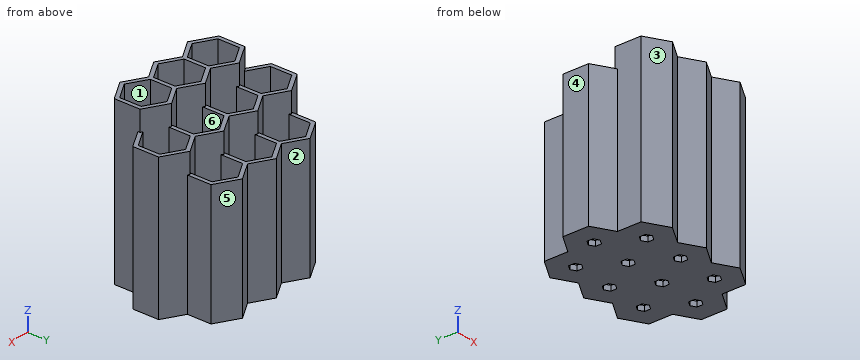
from build123d import *

# Parameters (mm, degrees)
F3_DEPTH = 101.6
F4_DEPTH = 88.9
F5_DEPTH = 76.2
F7_DEPTH = 3.175


with BuildPart() as f3:
    # F1 (on Top) → F3 (new body)
    with BuildSketch(Plane.XY):
        Polygon((0, -5.911706), (-12.620625, -13.198227), (-25.24125, -5.911706), (-39.0525, -13.885635), (-39.0525, -29.833493), (-25.24125, -37.807422), (-12.620625, -30.5209), (0, -37.807422), (12.620625, -30.5209), (25.24125, -37.807422), (39.0525, -29.833493), (39.0525, -13.885635), (25.24125, -5.911706), (12.620625, -13.198227), align=None)
        Polygon((0, -35.057791), (-11.43, -28.458677), (-11.43, -15.26045), (0, -8.661337), (11.43, -15.26045), (11.43, -28.458677), align=None, mode=Mode.SUBTRACT)
        Polygon((-25.24125, -35.057791), (-36.67125, -28.458677), (-36.67125, -15.26045), (-25.24125, -8.661337), (-13.81125, -15.26045), (-13.81125, -28.458677), align=None, mode=Mode.SUBTRACT)
        Polygon((13.81125, -28.458677), (13.81125, -15.26045), (25.24125, -8.661337), (36.67125, -15.26045), (36.67125, -28.458677), (25.24125, -35.057791), align=None, mode=Mode.SUBTRACT)
    extrude(amount=F3_DEPTH)

    # F0 (on Top) → F4 (join)
    with BuildSketch(Plane.XY):
        Polygon((-26.431875, -6.599114), (-24.050625, -6.599114), (-24.050625, 6.599114), (-12.620625, 13.198227), (-1.190625, 6.599114), (-1.190625, -6.599114), (1.190625, -6.599114), (1.190625, 6.599114), (12.620625, 13.198227), (24.050625, 6.599114), (24.050625, -6.599114), (26.431875, -6.599114), (26.431875, 6.599114), (37.861875, 13.198227), (49.291875, 6.599114), (49.291875, -6.599114), (37.861875, -13.198227), (39.0525, -15.26045), (51.673125, -7.973929), (51.673125, 7.973929), (37.861875, 15.947858), (25.24125, 8.661337), (12.620625, 15.947858), (0, 8.661337), (-12.620625, 15.947858), (-25.24125, 8.661337), (-37.861875, 15.947858), (-51.673125, 7.973929), (-51.673125, -7.973929), (-39.0525, -15.26045), (-37.861875, -13.198227), (-49.291875, -6.599114), (-49.291875, 6.599114), (-37.861875, 13.198227), (-26.431875, 6.599114), align=None)
    extrude(amount=F4_DEPTH)

    # F2 (on Top) → F5 (join)
    with BuildSketch(Plane.XY):
        Polygon((-13.81125, 15.26045), (-11.43, 15.26045), (-11.43, 28.458677), (0, 35.057791), (11.43, 28.458677), (11.43, 15.26045), (13.81125, 15.26045), (13.81125, 28.458677), (25.24125, 35.057791), (36.67125, 28.458677), (36.67125, 15.26045), (39.0525, 15.26045), (39.0525, 29.833493), (25.24125, 37.807422), (12.620625, 30.5209), (0, 37.807422), (-12.620625, 30.5209), (-25.24125, 37.807422), (-39.0525, 29.833493), (-39.0525, 15.26045), (-36.67125, 15.26045), (-36.67125, 28.458677), (-25.24125, 35.057791), (-13.81125, 28.458677), align=None)
    extrude(amount=F5_DEPTH)

    # F6 (on Top) → F7 (join)
    with BuildSketch(Plane.XY):
        Polygon((-49.291875, 6.599114), (-49.291875, -6.599114), (-37.861875, -13.198227), (-26.431875, -6.599114), (-26.431875, 6.599114), (-37.861875, 13.198227), align=None)
        Polygon((-37.861875, -3.666174), (-41.036875, -1.833087), (-41.036875, 1.833087), (-37.861875, 3.666174), (-34.686875, 1.833087), (-34.686875, -1.833087), align=None, mode=Mode.SUBTRACT)
        Polygon((-24.050625, 6.599114), (-24.050625, -6.599114), (-12.620625, -13.198227), (-1.190625, -6.599114), (-1.190625, 6.599114), (-12.620625, 13.198227), align=None)
        Polygon((-15.795625, -1.833087), (-15.795625, 1.833087), (-12.620625, 3.666174), (-9.445625, 1.833087), (-9.445625, -1.833087), (-12.620625, -3.666174), align=None, mode=Mode.SUBTRACT)
        Polygon((-13.81125, -28.458677), (-13.81125, -15.26045), (-25.24125, -8.661337), (-36.67125, -15.26045), (-36.67125, -28.458677), (-25.24125, -35.057791), align=None)
        Polygon((-28.41625, -23.692651), (-28.41625, -20.026477), (-25.24125, -18.19339), (-22.06625, -20.026477), (-22.06625, -23.692651), (-25.24125, -25.525738), align=None, mode=Mode.SUBTRACT)
        Polygon((-36.67125, 28.458677), (-36.67125, 15.26045), (-25.24125, 8.661337), (-13.81125, 15.26045), (-13.81125, 28.458677), (-25.24125, 35.057791), align=None)
        Polygon((-25.24125, 18.19339), (-28.41625, 20.026477), (-28.41625, 23.692651), (-25.24125, 25.525738), (-22.06625, 23.692651), (-22.06625, 20.026477), align=None, mode=Mode.SUBTRACT)
        Polygon((-11.43, 28.458677), (-11.43, 15.26045), (0, 8.661337), (11.43, 15.26045), (11.43, 28.458677), (0, 35.057791), align=None)
        Polygon((-3.175, 20.026477), (-3.175, 23.692651), (0, 25.525738), (3.175, 23.692651), (3.175, 20.026477), (0, 18.19339), align=None, mode=Mode.SUBTRACT)
        Polygon((13.81125, 28.458677), (13.81125, 15.26045), (25.24125, 8.661337), (36.67125, 15.26045), (36.67125, 28.458677), (25.24125, 35.057791), align=None)
        Polygon((25.24125, 25.525738), (28.41625, 23.692651), (28.41625, 20.026477), (25.24125, 18.19339), (22.06625, 20.026477), (22.06625, 23.692651), align=None, mode=Mode.SUBTRACT)
        Polygon((24.050625, -6.599114), (24.050625, 6.599114), (12.620625, 13.198227), (1.190625, 6.599114), (1.190625, -6.599114), (12.620625, -13.198227), align=None)
        Polygon((12.620625, -3.666174), (9.445625, -1.833087), (9.445625, 1.833087), (12.620625, 3.666174), (15.795625, 1.833087), (15.795625, -1.833087), align=None, mode=Mode.SUBTRACT)
        Polygon((26.431875, 6.599114), (26.431875, -6.599114), (37.861875, -13.198227), (49.291875, -6.599114), (49.291875, 6.599114), (37.861875, 13.198227), align=None)
        Polygon((34.686875, 1.833087), (37.861875, 3.666174), (41.036875, 1.833087), (41.036875, -1.833087), (37.861875, -3.666174), (34.686875, -1.833087), align=None, mode=Mode.SUBTRACT)
        Polygon((36.67125, -28.458677), (36.67125, -15.26045), (25.24125, -8.661337), (13.81125, -15.26045), (13.81125, -28.458677), (25.24125, -35.057791), align=None)
        Polygon((22.06625, -20.026477), (25.24125, -18.19339), (28.41625, -20.026477), (28.41625, -23.692651), (25.24125, -25.525738), (22.06625, -23.692651), align=None, mode=Mode.SUBTRACT)
        Polygon((-11.43, -15.26045), (-11.43, -28.458677), (0, -35.057791), (11.43, -28.458677), (11.43, -15.26045), (0, -8.661337), align=None)
        Polygon((-3.175, -23.692651), (-3.175, -20.026477), (0, -18.19339), (3.175, -20.026477), (3.175, -23.692651), (0, -25.525738), align=None, mode=Mode.SUBTRACT)
    extrude(amount=F7_DEPTH)


solid = f3.part
Source: CAD feature listing. Evaluate the final solid. Frame: model axes, mm. Face numbers are marked on the shaded views. A direction names the side the tool comes from. Coordinates: 2 decimals unless noted, no trailing zeros. Loops run counter-clockwise (first coordinate to the right, second up) from the corner with the lowest first, then second, coordinate; pieces in that order, holes last. Notation, with made-up numbers: (89.5, 46.25) - (112.5, 46.25) arc R28 cw to (112.5, 69.25) - close; hole circle Ø3 at (76, -31). An arc over 180 degrees is marked (long way). One line per item, written item: value. Start each with the question number.
1. Section A-A (z = 92). State how many separate pieces and enclosed holes the cut face has, and give its area (3 significant figures).
2. Section C-C (x = 30). Return the cut outline in (y, z) (3 decimals), and give its area (3 significant figures).
3. Contact query for flat-ended pins moving along their axis: P1, Ø1.6, axis at y = 22, z = 1.5, coming from the +X side; P2, Ø1.5, axis at x = -30.5, y = -28, coming from the -Z side; P3, Ø1.5, axis at x = -39.5, y = 24, coming from the +Z side; P4, Ø10.5, axis at y = -21.5, z = 56.5, coming from the -X side. Output: stop coordinate, or through.
4. Mould query, pull axis X, two halves, no side actions, for the marked faces 4, 5 and 6. Classes: pulls with the +X half, pulls with the -X half, needs draft (parallel to the pull), parting line crosses it, or undercut.
5. Ray query, L1, parallel to X at y = 22, z = 13.5; L2, parallel to X at y = 4.5, z = 35; L3, parallel to Y at x = 11, z = 26. Return the intervals inside material, ascending.
6. Set-up query: the marked faces 1, 2 and 3. Return all of +Z, -Z, +X, -X, +Y, -Y with unobstructed straight access to the full face (end or side cutting, diameter ignored); none if empty.
Verdict:
1. separate pieces: 1
1. enclosed holes: 3
1. area: 545 mm2
2. outline: (-35.06, 0) - (35.06, 0) - (35.06, 76.2) - (32.31, 76.2) - (32.31, 3.175) - (11.409, 3.175) - (11.409, 88.9) - (8.659, 88.9) - (8.659, 3.175) - (-8.659, 3.175) - (-8.659, 101.6) - (-11.409, 101.6) - (-11.409, 3.175) - (-32.31, 3.175) - (-32.31, 101.6) - (-35.06, 101.6) - close
2. area: 1,200 mm2
3. P1: stops at x = 39.05
3. P2: stops at z = 0
3. P3: stops at z = 76.2
3. P4: stops at x = -39.05
4. face 4: pulls with the -X half
4. face 5: pulls with the +X half
4. face 6: undercut
5. L1: x = -39.05 to -36.67, -13.81 to -11.43, 11.43 to 13.81, 36.67 to 39.05
5. L2: x = -51.67 to -49.29, -26.43 to -24.05, -1.19 to 1.19, 24.05 to 26.43, 49.29 to 51.67
5. L3: y = -31.46 to -28.71, -15.01 to -12.26, 12.26 to 15.01, 28.71 to 31.46
6. face 1: +Z
6. face 2: +Z, -Z, +Y
6. face 3: +Z, -Z, -X, -Y
